```python
from build123d import *

# Parameters (mm, degrees)
ESQUISSE1_W             = 220
ESQUISSE1_H             = 4
BOSS_EXTRU_1_DEPTH      = 3
ESQUISSE2_R             = 1
ENL_V_MAT_EXTRU_1_DEPTH = 6
CONG_1_R                = 1
CONG_2_R                = 1


with BuildPart() as part:
    # Esquisse1 → Boss.-Extru.1 (new body)
    with BuildSketch(Plane.XY):
        with Locations((-110, 2)):
            Rectangle(ESQUISSE1_W, ESQUISSE1_H)
    extrude(amount=BOSS_EXTRU_1_DEPTH)

    # Esquisse2 → Enlèv. mat.-Extru.1 (cut)
    with BuildSketch(Plane.XY.offset(3)):
        with Locations((-2, 2)):
            Circle(ESQUISSE2_R)
        with Locations((-213.150378979, 2)):
            Circle(ESQUISSE2_R)
    extrude(amount=-ENL_V_MAT_EXTRU_1_DEPTH, mode=Mode.SUBTRACT)

    # Congé1
    cong_1_edges = [part.edges().sort_by_distance(p)[0] for p in [
        (0, 4, 1.5),
    ]]
    fillet(cong_1_edges, radius=CONG_1_R)

    # Congé2
    cong_2_edges = [part.edges().sort_by_distance(p)[0] for p in [
        (0, 0, 1.5),
    ]]
    fillet(cong_2_edges, radius=CONG_2_R)


solid = part.part
```
Verification items for the finished model (mm, model axes). Give positions to 0.01 mm unless a question says otherwise; leave off trailing zeros. Order: outer loops, then holes, each group sorted by start corner. A loop starts at its lowest first (then second) coordinate and runs counter-clockwise, first axis right, second up. Notation, with made-up numbers: (50, 64.25) -> (86, 64.25) arc R17 cw to (86, 94.25) -> close; hole circle Ø9 at (-31, 26). An arc over 180 degrees is marked (long way). Use a Markdown table: item, result.
1) Section check A-A, the plane y = 2. Record the boundary of the cut face in (x, z).
Results:
| item | result |
|---|---|
| outline | (-220, 0) -> (-214.15, 0) -> (-214.15, 3) -> (-220, 3) -> close; (-212.15, 0) -> (-3, 0) -> (-3, 3) -> (-212.15, 3) -> close; (-1, 0) -> (0, 0) -> (0, 3) -> (-1, 3) -> close |
2) Material ranges on probe 1 along X at (y, z) = (2.05, 2.55); probe 2 along Y at (x, z) = (-2, 0.95); probe 3 along X at (y, z) = (2.35, 1.8), recorded low to high.
Results:
| item | result |
|---|---|
| probe 1 | -220 to -214.15, -212.15 to -3, -1 to 0 |
| probe 2 | 0 to 1, 3 to 4 |
| probe 3 | -220 to -214.09, -212.21 to -2.94, -1.06 to 0 |
3) Depth check by flat-ended pin: pin 1 Ø1.8 at (x, y) = (-213.15, 2) entering from -Z. Enter the tip coordinate at first touch or a pass-through.
Results:
| item | result |
|---|---|
| pin 1 | through |
